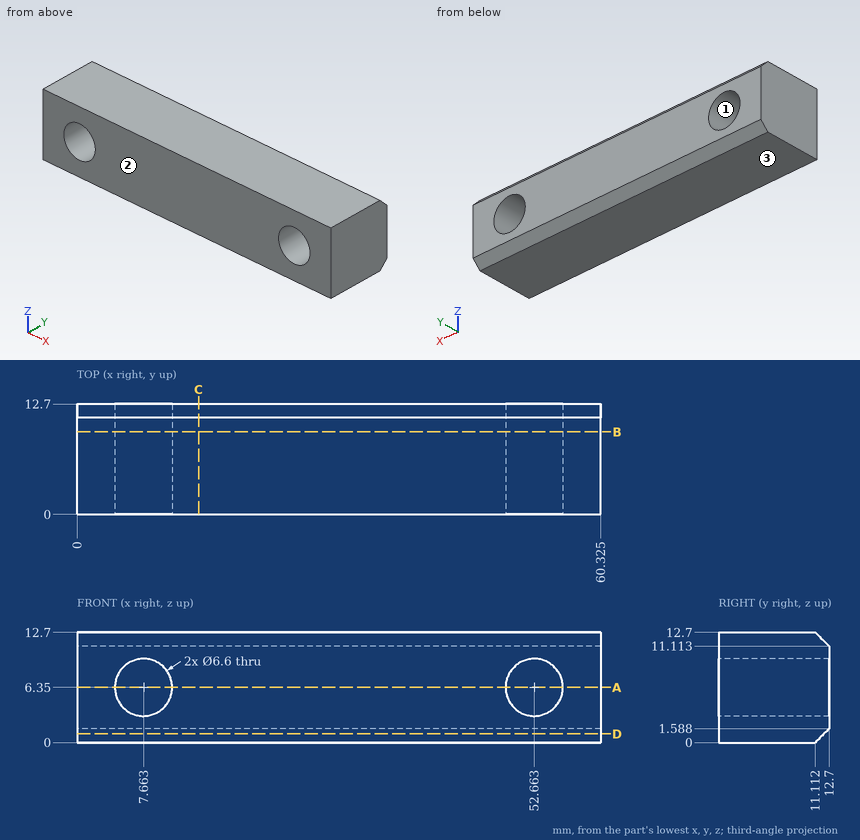
Geometry: see drawing. Coordinates: mm, zero at the bounding-box minimum. Round coordinates to 2 decimals unless told otherwise and drop trailing zeros. Write each loop counter-clockwise with the first axis right and the second up, starting at its lowest first coordinate (ties: lowest second). Pieces come first, ordered by that corner, then holes.
1) Cut plane D-D (z = 1). Return the cut outline in (x, y) (1 decimal), then the cut area to 3 significant figures.
2) Cut plane A-A (z = 6.35). Return the cut outline in (x, y) (1 decimal).
3) Draft query along Z for the marked faces 1, 2 and 3. Return one class per face: pulls with the +Z half, pulls with the -Z half, needs draft (parallel to the pull), parting line crosses it, or undercut.
4) Cut plane C-C (x = 14). Return the cut outline in (y, z).
5) Ray query, L1, parallel to X at y = 3.5, z = 6.5 (1 decimal); L2, parallel to X at y = 3, z = 9.25 (1 decimal); L3, parallel to Z at x = 7, y = 8.5. Return the intervals inside material, ascending.
6) Cut plane B-B (y = 9.5). Count the separate pieces of the cut face and the enclosed holes in it, then the cut area to 3 significant figures.
Geometry says:
1. outline: (0, 0) - (60.3, 0) - (60.3, 12.1) - (0, 12.1) - close
1. area: 731 mm2
2. outline: (0, 0) - (4.4, 0) - (4.4, 12.7) - (0, 12.7) - close; (11, 0) - (49.4, 0) - (49.4, 12.7) - (11, 12.7) - close; (56, 0) - (60.3, 0) - (60.3, 12.7) - (56, 12.7) - close
3. face 1: undercut
3. face 2: needs draft
3. face 3: pulls with the -Z half
4. outline: (0, 0) - (11.11, 0) - (12.7, 1.59) - (12.7, 11.11) - (11.11, 12.7) - (0, 12.7) - close
5. L1: x = 0 to 4.4, 11 to 49.4, 56 to 60.3
5. L2: x = 0 to 6.1, 9.2 to 51.1, 54.2 to 60.3
5. L3: z = 0 to 3.12, 9.58 to 12.7
6. separate pieces: 1
6. enclosed holes: 2
6. area: 698 mm2
